Work out the finished part from the listing and answer in its coordinate system (mm). A direction names the side the tool comes from. Give positions to 0.01 mm unless a question says otherwise; leave off trailing zeros. Write each loop counter-clockwise with the first axis right and the second up, starting at its lowest first coordinate (ties: lowest second). Pieces come first, ordered by that corner, then holes. Notation, with made-up numbers: (-6, 83.5) - (36, 83.5) arc R19 ccw to (36, 118.5) - close; hole circle Ø11 at (13.5, -8.5). An arc over 180 degrees is marked (long way). Write each question's results on one line, items separated by ' | '. Start each with the question number.
Autodesk Inventor part; units mm, degrees
ref_plane "YZ Plane" through (0, 0, 0) normal (1, 0, 0) x (0, 1, 0)
ref_plane "XZ Plane" through (0, 0, 0) normal (0, 1, 0) x (-1, 0, 0)
ref_plane "XY Plane" through (0, 0, 0) normal (0, 0, 1) x (1, 0, 0)
sketch "Skizze3" plane through (0, 0, 0) normal (0, 0, 1) x (1, 0, 0)
  line L0 (0, 0) -> (30, 0)
  line L1 (30, 0) -> (30, 48)
  line L2 (30, 48) -> (0, 48)
  line L3 (0, 48) -> (0, 0)
  dimension "d14" = 30
  dimension "d15" = 48
extrude "Extrusion3" add sketch "Skizze3" along normal blind 10
sketch "Skizze4" plane through (0, 0, 0) normal (-1, 0, 0) x (0, 0, 1)
  line L0 (10, 0) -> (10, 48)
  arc A0 (10, 21.5) -> (10, 6.5) centre (10, 14) ccw
  line L1 (10, 21.5) -> (10, 6.5)
  point P0 (0, 0)
  dimension "d18" = 7.5
  dimension "d19" = 14
extrude "Extrusion4" cut sketch "Skizze4" against normal up to next
sketch "Skizze5" plane through (0, 0, 10) normal (0, 0, 1) x (1, 0, 0)
  line L0 (0, 40.7) -> (30, 40.7)
  line L1 (30, 40.7) -> (30, 38.7)
  line L2 (0, 38.7) -> (0, 40.7)
  line L3 (30, 38.7) -> (28, 38.7)
  line L4 (0, 38.7) -> (2, 38.7)
  line L5 (30, 48) -> (0, 48)
  line L6 (26, 36.7) -> (26, 33.7)
  line L7 (24, 31.7) -> (6, 31.7)
  line L8 (4, 33.7) -> (4, 36.7)
  line L9 (0, 21.5) -> (30, 21.5)
  arc A0 (4, 36.7) -> (2, 38.7) centre (2, 36.7) ccw
  arc A1 (4, 33.7) -> (6, 31.7) centre (6, 33.7) ccw
  arc A2 (24, 31.7) -> (26, 33.7) centre (24, 33.7) ccw
  arc A3 (28, 38.7) -> (26, 36.7) centre (28, 36.7) ccw
  line L10 (7.5, 36.7) -> (12, 36.7) construction
  line L11 (7.5, 34.7) -> (12, 34.7)
  line L12 (12, 38.7) -> (7.5, 38.7)
  arc A4 (7.5, 38.7) -> (7.5, 34.7) centre (7.5, 36.7) ccw
  arc A5 (12, 34.7) -> (12, 38.7) centre (12, 36.7) ccw
  line L13 (18, 36.7) -> (22.5, 36.7) construction
  line L14 (18, 34.7) -> (22.5, 34.7)
  line L15 (22.5, 38.7) -> (18, 38.7)
  arc A6 (18, 38.7) -> (18, 34.7) centre (18, 36.7) ccw
  arc A7 (22.5, 34.7) -> (22.5, 38.7) centre (22.5, 36.7) ccw
  line L16 (30, 21.5) -> (30, 48)
  line L17 (0, 48) -> (0, 21.5)
  point P0 (26, 38.7)
  point P1 (4, 38.7)
  point P2 (26, 31.7)
  point P3 (4, 31.7)
  point P4 (9.75, 36.7)
  point P5 (20.25, 36.7)
  dimension "d22" = 2
  dimension "d28" = 4
  dimension "d29" = 4
  dimension "d30" = 2
  dimension "d34" = 7
  dimension "d48" = 2
  dimension "d83" = 7.3
  dimension "d84" = 4.5
  dimension "d85" = 4
  dimension "d86" = 3.5
  dimension "d87" = 5
  dimension "d88" = 4.5
  dimension "d89" = 4
  dimension "d90" = 3.5
  dimension "d91" = 5
extrude "Extrusion5" cut sketch "Skizze5" against normal blind 3.5 contours L0 L1 L3 A3 L6 A2 L7 A1 L8 A0 L4 L2
sketch "Skizze6" plane through (0, 0, 10) normal (0, 0, 1) x (1, 0, 0)
  line L0 (0, 48) -> (0, 0)
  line L1 (30, 0) -> (30, 48)
  circle A0 centre (15, 44.2) radius 3.05
  line L2 (0, 40.7) -> (30, 40.7)
  dimension "d43" = 6.1
  dimension "d44" = 15
  dimension "d45" = 3.5
extrude "Extrusion6" cut sketch "Skizze6" against normal up to next
sketch "Skizze7" plane through (0, 0, 10) normal (0, 0, 1) x (1, 0, 0)
  circle A0 centre (5, 25) radius 1.55
  circle A1 centre (25, 25) radius 1.55
  circle A2 centre (15, 4) radius 1.55
  line L0 (0, 6.5) -> (0, 21.5)
  line L1 (30, 21.5) -> (30, 6.5)
  line L2 (0, 0) -> (30, 0)
  line L3 (0, 6.5) -> (0, 0)
  line L4 (0, 21.5) -> (30, 21.5)
  point P0 (0, 38.7)
  point P1 (30, 38.7)
  dimension "d49" = 3.1
  dimension "d50" = 3.1
  dimension "d51" = 3.1
  dimension "d53" = 5
  dimension "d54" = 5
  dimension "d55" = 4
  dimension "d74" = 15
  dimension "d75" = 3.5
  dimension "d76" = 3.5
extrude "Extrusion7" cut sketch "Skizze7" against normal up to next
sketch "Skizze8" plane through (30, 0, 0) normal (1, 0, 0) x (0, 0, -1)
  arc A0 (-10, 6.5) -> (-10, 21.5) centre (-10, 14) ccw
  arc A1 (-10, 9) -> (-10, 19) centre (-10, 14) ccw
  line L0 (-10, 19) -> (-10, 21.5)
  line L1 (-10, 9) -> (-10, 6.5)
  arc A2 (-10, 6.5) -> (-10, 21.5) centre (-10, 14) ccw
  point P0 (0, 0)
  dimension "d59" = 5
extrude "Extrusion8" add sketch "Skizze8" against normal blind 3
sketch "Skizze10" plane through (0, 0, 0) normal (-1, 0, 0) x (0, 0, 1)
  arc A0 (10, 19) -> (10, 9) centre (10, 14) ccw
  arc A1 (10, 21.5121) -> (10, 6.4879) centre (10, 14) ccw
  arc A2 (10, 19) -> (10, 9) centre (10, 14) ccw
  line L0 (10, 19) -> (10, 21.5121)
  line L1 (10, 6.5) -> (10, 21.5)
  line L2 (10, 9) -> (10, 6.4879)
  point P0 (0, 0)
  point P1 (10, 38.7)
extrude "Extrusion9" add sketch "Skizze10" against normal blind 3 contours A0 L1 L2 A1 L0
fillet "Rundung1" radius 2 4 edges at (30, 0, 5) (0, 0, 5) (0, 48, 5) (30, 48, 5)
sketch "Skizze14" plane through (0, 0, 0) normal (0, 0, -1) x (-1, 0, 0)
  circle A0 centre (-5, 25) radius 1.55
  circle A1 centre (-5, 25) radius 2.9 construction
  circle A2 centre (-25, 25) radius 1.55
  circle A3 centre (-25, 25) radius 2.9 construction
  line L0 (-7.9, 26.6743) -> (-5, 28.3486)
  line L1 (-5, 28.3486) -> (-2.1, 26.6743)
  line L2 (-2.1, 26.6743) -> (-2.1, 23.3257)
  line L3 (-2.1, 23.3257) -> (-5, 21.6514)
  line L4 (-5, 21.6514) -> (-7.9, 23.3257)
  line L5 (-7.9, 23.3257) -> (-7.9, 26.6743)
  line L6 (-22.1, 23.3257) -> (-25, 21.6514)
  line L7 (-25, 21.6514) -> (-27.9, 23.3257)
  line L8 (-27.9, 23.3257) -> (-27.9, 26.6743)
  line L9 (-27.9, 26.6743) -> (-25, 28.3486)
  line L10 (-25, 28.3486) -> (-22.1, 26.6743)
  line L11 (-22.1, 26.6743) -> (-22.1, 23.3257)
  circle A4 centre (-15, 4) radius 2.9 construction
  line L12 (-16.6743, 1.1) -> (-18.3486, 4)
  line L13 (-18.3486, 4) -> (-16.6743, 6.9)
  line L14 (-16.6743, 6.9) -> (-13.3257, 6.9)
  line L15 (-13.3257, 6.9) -> (-11.6514, 4)
  line L16 (-11.6514, 4) -> (-13.3257, 1.1)
  line L17 (-13.3257, 1.1) -> (-16.6743, 1.1)
  point P0 (0, 0)
  point P1 (-7.9, 25)
  point P2 (-22.1, 25)
  point P3 (-15, 1.1)
  dimension "d92" = 5.8
  dimension "d95" = 5.8
  dimension "d98" = 5.8
  dimension "d99" = 0
  dimension "d100" = 0
extrude "Extrusion13" cut sketch "Skizze14" against normal blind 3.2
properties part number "Lagerblock XY" material "ABS-Kunststoff"
Q1. A cutting plane is placed at B-B, the plane y = 44.2. Write down the section's boundary in (x, z), and give its area (3 significant figures).
Q2. A tool of negligible diameter and unlimited length cuts with its end or side. For faces 5 (the flat face through (1, 38.7, 8)), 6 (the flat face through (23.8, 23.6, 3.2)), 7 (the flat face through (27, 14.1, 4.6)), from which of +Z, -Z, +X, -X, +Y, -Y can it reach the whole face along a straight path? Write none if from no direction.
Q3. A cutting plane is placed at A-A, the plane x = 15. Write down the section's boundary in (y, z), and give its area (3 significant figures).
Q4. A cutting plane is placed at C-C, the plane y = 14. Write down the section's boundary in (x, z), and give its area (3 significant figures).
Q5. Given pin 1 (6 mm diameter, centred on x = 7.5, z = 8, fed in from -Y); pin 2 (1 mm diameter, centred on x = 1, z = 8.5, fed in from +Y); pin 3 (5 mm diameter, centred on x = 5, y = 25, fed in from -Z), each flat-ended and moving along its own axis, determine where each tip first touches the part or whether it passes through.
Q6. A cutting plane is placed at D-D, the plane x = 9. Write down the section's boundary in (y, z).
Q7. Consider L1, parallel to X at y = 25, z = 5.5; L2, parallel to X at y = 15, z = 3.25; L3, parallel to Y at x = 25, z = 5.75. Determine where each line is inside the solid, lowest interval first.
Q8. The mould has two halves that part along Y. Classify faces 1 (the cylindrical face through (0.57, 0.6, 5.07)), 2 (the cylindrical face through (14, 36.7, 8.3)), 3 (the flat face through (15, 48, 5)), 4 (the cylindrical face through (16, 36.7, 8.3)): pulls with the +Y half, pulls with the -Y half, needs draft (parallel to the pull), parting line crosses it, or undercut.
Result:
1) outline: (0, 0) - (11.95, 0) - (11.95, 10) - (0, 10) - close; (18.05, 0) - (30, 0) - (30, 10) - (18.05, 10) - close | area: 239 mm2
2) face 5: +Z, +X, -X | face 6: -Z | face 7: +Z
3) outline: (0, 0) - (1.1, 0) - (1.1, 3.2) - (2.45, 3.2) - (2.45, 10) - (0, 10) - close; (5.55, 3.2) - (6.9, 3.2) - (6.9, 0) - (41.15, 0) - (41.15, 10) - (40.7, 10) - (40.7, 6.5) - (31.7, 6.5) - (31.7, 10) - (21.5, 10) arc R7.5 cw to (6.5, 10) - (5.55, 10) - close; (47.25, 0) - (48, 0) - (48, 10) - (47.25, 10) - close | area: 260 mm2
4) outline: (0, 0) - (30, 0) - (30, 5) - (27, 5) - (27, 2.5) - (3, 2.5) - (3, 5) - (0, 5) - close | area: 90.0 mm2
5) pin 1: stops at y = 0 | pin 2: stops at y = 47.94 | pin 3: stops at z = 3.2
6) outline: (0, 0) - (48, 0) - (48, 10) - (40.7, 10) - (40.7, 6.5) - (38.7, 6.5) - (38.7, 10) - (34.7, 10) - (34.7, 6.5) - (31.7, 6.5) - (31.7, 10) - (21.5, 10) arc R7.5 cw to (6.5, 10) - (0, 10) - close
7) L1: x = 0 to 3.45, 6.55 to 23.45, 26.55 to 30 | L2: x = 0 to 3, 27 to 30 | L3: y = 0 to 7.82, 20.18 to 23.45, 26.55 to 48
8) face 1: pulls with the -Y half | face 2: undercut | face 3: pulls with the +Y half | face 4: undercut
